```python
from build123d import *
from build123d import SkipClean  # not in build123d's __all__

# Parameters (mm, degrees)
F1_DEPTH = 25.4
F2_DEPTH = 25.4
F3_DEPTH = 12.7
F4_R     = 12.69999
F5_SIZE  = 2.54


# Not quite as in the source:
# - a fillet or chamfer is up to 0.001 mm smaller than in the source, because OpenCascade refuses the exact size
# - after a boolean that leaves OpenCascade's solid faulty, fix() repairs it


with BuildPart() as f1:
    # F0 (on Front) → F1 (new body)
    with BuildSketch(Plane.XZ):
        with BuildLine():
            ThreePointArc((-51.8046888554, -8.5958305632), (-36.6155359926, 3.0241505339), (-30.8559403173, 21.2604161342))
            ThreePointArc((-30.8559403173, 21.2604161342), (-35.9540680262, 38.515566188), (-49.6112287191, 50.2293645183))
            ThreePointArc((-49.6112287191, 50.2293645183), (-94.3338910639, 22.443480552), (-51.8046888554, -8.5958305632))
        make_face()
        with BuildLine():
            ThreePointArc((-49.6112287191, 50.2293645183), (-35.9540680262, 38.515566188), (-30.8559403173, 21.2604161342))
            ThreePointArc((-30.8559403173, 21.2604161342), (-36.6155359926, 3.0241505339), (-51.8046888554, -8.5958305632))
            Line((-51.8046888554, -8.5958305632), (-7.5207185378, 7.4250143868))
            ThreePointArc((-7.5207185378, 7.4250143868), (-24.5323994212, 19.8407388329), (-6.6433344833, 30.9550924194))
            Line((-6.6433344833, 30.9550924194), (-49.6112287191, 50.2293645183))
        make_face()
        with BuildLine():
            ThreePointArc((0.8587808774, 19.3675130658), (-1.1804702061, 26.2695730873), (-6.6433344833, 30.9550924194))
            ThreePointArc((-6.6433344833, 30.9550924194), (-24.5323994212, 19.8407388329), (-7.5207185378, 7.4250143868))
            ThreePointArc((-7.5207185378, 7.4250143868), (-1.4450573927, 12.0730068257), (0.8587808774, 19.3675130658))
        make_face()
    extrude(amount=F1_DEPTH)

    # F0 (on Front) → F2 (join)
    with BuildSketch(Plane.XZ):
        with BuildLine():
            ThreePointArc((-51.8046888554, -8.5958305632), (-36.6155359926, 3.0241505339), (-30.8559403173, 21.2604161342))
            ThreePointArc((-30.8559403173, 21.2604161342), (-35.9540680262, 38.515566188), (-49.6112287191, 50.2293645183))
            ThreePointArc((-49.6112287191, 50.2293645183), (-94.3338910639, 22.443480552), (-51.8046888554, -8.5958305632))
        make_face()
    with SkipClean():  # cleaning this boolean's faces spoils the solid; the shape is the same uncleaned
        extrude(amount=-F2_DEPTH)

    # F0 (on Front) → F3 (join)
    with BuildSketch(Plane.XZ):
        with BuildLine():
            ThreePointArc((0.8587808774, 19.3675130658), (-1.1804702061, 26.2695730873), (-6.6433344833, 30.9550924194))
            ThreePointArc((-6.6433344833, 30.9550924194), (-24.5323994212, 19.8407388329), (-7.5207185378, 7.4250143868))
            ThreePointArc((-7.5207185378, 7.4250143868), (-1.4450573927, 12.0730068257), (0.8587808774, 19.3675130658))
        make_face()
    extrude(amount=-F3_DEPTH)

    add(f1.part.fix(), mode=Mode.REPLACE)

    # F4 (radius 12.7 in the source; OpenCascade refuses exactly that, so slightly less here)
    f4_edges = [f1.edges().sort_by_distance(p)[0] for p in [
        (-16.16172, 12.7, 31.310012),
    ]]
    fillet(f4_edges, radius=F4_R)

    # F5
    f5_edges = [f1.edges().sort_by_distance(p)[0] for p in [
        (-73.407192, 25.4, 51.116663),
    ]]
    chamfer(f5_edges, length=F5_SIZE)


solid = f1.part
```
The model under review builds one solid part; all positions refer to its coordinate system, in mm. Round coordinates to 2 decimals unless told otherwise and drop trailing zeros. Order: outer loops, then holes, each group sorted by start corner. A loop starts at its lowest first (then second) coordinate and runs counter-clockwise, first axis right, second up.
Item 1: Draft analysis for pull direction X (two halves, no side actions). For faces 1 (the flat face through (-27.83, -12.52, 40.46)), 2 (the flat face through (-47, -25.4, 22)), 3 (the flat face through (-28, 0, 19)), state which applies: released by +X, released by -X, zero draft, split by the parting line, or undercut.
Working result:
face 1: released by +X
face 2: zero draft
face 3: undercut
Item 2: For pin 1 (4 mm diameter, centred on y = -12.5, z = -1.5, fed in from -X); pin 2 (4 mm diameter, centred on x = -26.5, y = -13, fed in from +Z); pin 3 (1.5 mm diameter, centred on x = -27.5, z = 22, fed in from +Y), all flat-tipped, find the tip position at first contact; note any pin that passes through.
Working result:
pin 1: stops at x = -86.63
pin 2: stops at z = 40.76
pin 3: stops at y = 0
Item 3: Add section B-B, the plane y = 16. State the section outline as (x, z) points.
Working result:
outline: circle Ø63.5 at (-62.61, 21.26)
Item 4: To check wall thickness, follow probe 1 along Y at (x, z) = (-26.5, 14); probe 2 along Y at (x, z) = (-10.5, 16). State the ranges of each line that lie inside material, in increasing order.
Working result:
probe 1: y = -25.4 to 0
probe 2: y = -25.4 to 12.17
Item 5: Add section A-A, the plane y = -19. State the section outline as (x, z) points, and give its area (3 significant figures).
Working result:
outline: (-51.8, -8.6) - (-7.52, 7.43) arc R12.7 ccw to (-6.64, 30.96) - (-49.61, 50.23) arc R31.75 ccw (long way) to start
area: 4,260 mm2
